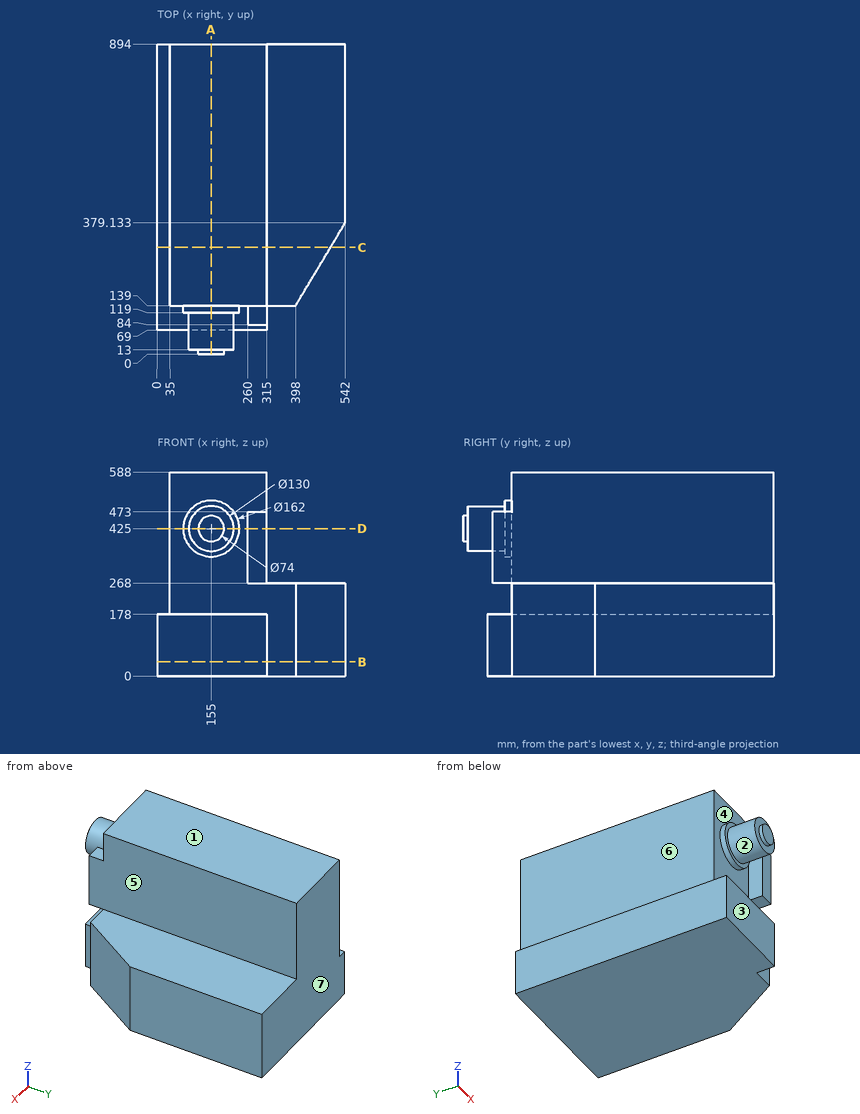
Can you work these out from the drawing? Everything is in mm from the part's minimum corner. A direction names the side the tool comes from. Round coordinates to 2 decimals unless told otherwise and drop trailing zeros. Loops run counter-clockwise (first coordinate to the right, second up) from the corner with the lowest first, then second, coordinate; pieces in that order, holes last. Notation, with made-up numbers: (34, 82.5) - (46, 82.5) arc R31 cw to (46, 109.5) - close; hole circle Ø1 at (43.25, -13.75). An arc over 180 degrees is marked (long way). Write item = value, one per line. Start each with the question number.
(1) If we section it at B-B (z = 41): Please give me the cut outline in (x, y).
(2) If we section it at A-A (x = 155): Please give me the cut outline in (y, z).
(3) If I drill on probe 1 along X at (y, z) = (725, 187); probe 2 along Y at (x, z) = (283.5, 364); probe 3 along Y at (x, z) = (120.5, 400), over which ranges is the centre line in solid material (lowest first)? Write a range as [from, to].
(4) For P1, Ø1, axis at y = 734, z = 348, coming from the +X side; P2, Ø2, axis at y = 296.5, z = 191.5, coming from the +X side; P3, Ø3, axis at x = 396.5, y = 486.5, coming from the +Z side, each with a flat end and sliding along its axis, tell me the tip position at first contact or that it passes through.
(5) If we section it at D-D (z = 425): Please give me the cut outline in (x, y), and give its area (3 significant figures).
(6) If we section it at C-C (y = 307.5): Please give me the cut outline in (x, z).
(7) If we mould it in two halves opening along Z, with no side actions, what happens to the marked faces 1, 2, 3 and 4? For each: released by +Z, released by -Z, zero draft, split by the parting line, or undercut.
(8) For the marked faces 5, 6 and 7, which set-ups out of +Z, -Z, +X, -X, +Y, -Y let a thin tool reach every point of the face, with its end or its side?
Ans:
q1.outline = (0, 69) - (315, 69) - (315, 139) - (398, 139) - (542, 379.13) - (542, 894) - (0, 894) - close
q2.outline = (0, 388) - (13, 388) - (13, 360) - (119, 360) - (119, 344) - (139, 344) - (139, 178) - (69, 178) - (69, 0) - (894, 0) - (894, 588) - (139, 588) - (139, 506) - (119, 506) - (119, 490) - (13, 490) - (13, 462) - (0, 462) - close
q3.probe_1 = [35, 542]
q3.probe_2 = [84, 894]
q3.probe_3 = [13, 894]
q4.P1 = 315
q4.P2 = 493.05
q4.P3 = 268
q5.outline = (35, 139) - (74, 139) - (74, 119) - (90, 119) - (90, 13) - (118, 13) - (118, 0) - (192, 0) - (192, 13) - (220, 13) - (220, 119) - (236, 119) - (236, 139) - (260, 139) - (260, 84) - (315, 84) - (315, 894) - (35, 894) - close
q5.area = 232,000 mm²
q6.outline = (0, 0) - (499.04, 0) - (499.04, 268) - (315, 268) - (315, 588) - (35, 588) - (35, 178) - (0, 178) - close
q7.face_1 = released by +Z
q7.face_2 = undercut
q7.face_3 = zero draft
q7.face_4 = undercut
q8.face_5 = +Z, +X, +Y, -Y
q8.face_6 = +Z, -X, +Y, -Y
q8.face_7 = +Z, -Z, +X, -X, +Y
